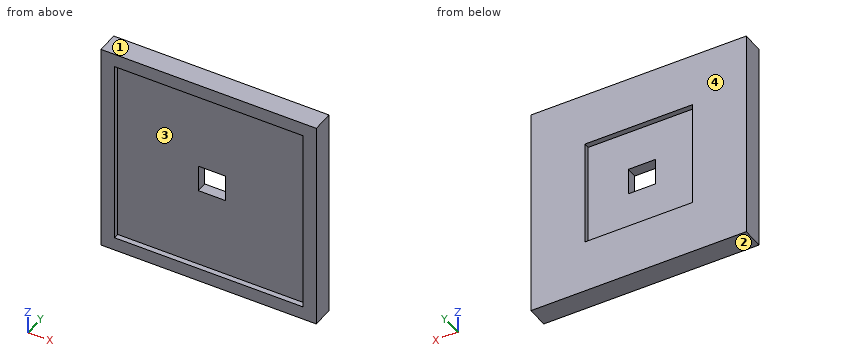
```python
from build123d import *

# Parameters (mm, degrees)
F0_W     = 101.6
F0_H     = 101.6
F1_DEPTH = 10.16
F2_W     = 88.9
F2_H     = 88.9
F3_DEPTH = 2.54
F4_W     = 50.8
F4_H     = 50.8
F5_DEPTH = 2.54
F6_W     = 12.7
F6_H     = 12.7
F7_DEPTH = 25.4


with BuildPart() as f1:
    # F0 (on Front) → F1 (new body)
    with BuildSketch(Plane.XZ):
        with Locations((4.06957, 6.01474)):
            Rectangle(F0_W, F0_H)
    extrude(amount=F1_DEPTH)

    # F2 (on face) → F3 (cut)
    with BuildSketch(Plane.XZ.offset(10.16)):
        with Locations((4.06957, 6.01474)):
            Rectangle(F2_W, F2_H)
    extrude(amount=-F3_DEPTH, mode=Mode.SUBTRACT)

    # F4 (on face) → F5 (cut)
    with BuildSketch(Plane(origin=(0, 0, 0), x_dir=(-1, 0, 0), z_dir=(0, 1, 0))):
        with Locations((-4.06957, 6.01474)):
            Rectangle(F4_W, F4_H)
    extrude(amount=-F5_DEPTH, mode=Mode.SUBTRACT)

    # F6 (on face) → F7 (cut)
    with BuildSketch(Plane(origin=(0, -2.54, 0), x_dir=(-1, 0, 0), z_dir=(0, 1, 0))):
        with Locations((-4.06957, 6.01474)):
            Rectangle(F6_W, F6_H)
    extrude(amount=-F7_DEPTH, mode=Mode.SUBTRACT)


solid = f1.part
```
The listing builds one solid part. Answer for the finished solid, in the listing's coordinates (mm). Face numbers are marked on the shaded views. Give positions to 0.01 mm unless a question says otherwise; leave off trailing zeros. Order: outer loops, then holes, each group sorted by start corner. A loop starts at its lowest first (then second) coordinate and runs counter-clockwise, first axis right, second up. Notation, with made-up numbers: M 47.5,61.5 L 101.5,61.5 A16 cw 101.5,83.5 Z; hole C 3.25,38.25 d3. An arc over 180 degrees is marked long. Put each result on its own line as item: value. Start each with the question number.
Item 1: The part is cut by section D-D, the plane x = -14. Determine the outline of the cut face in (y, z).
Item 2: The part is cut by section A-A, the plane y = -6.25. Determine the outline of the cut face in (x, z), and give its area (3 significant figures).
Item 3: For a pull along Z with two mould halves and no side action, classify the marked faces 1, 2, 3 and 4 as +Z half, -Z half, draft (parallel to the pull), parting line (faces both ways), or undercut.
Item 4: A flat-ended cylindrical pin translates along its axis: P1, Ø1.5, axis at x = -35, z = 35.5, coming from the -Y side. Find the tip coordinate at first contact, or state that the pin passes through.
Item 5: Find the intervals of material crossed by line 1 along X through (y, z) = (-8.5, -17.5); line 2 along Z through (x, y) = (32, -7.75); line 3 along X through (y, z) = (-2.25, -16), in increasing order.
Item 6: The part is cut by section B-B, the plane x = 4.5. Determine the outline of the cut face in (y, z), and give its area (3 significant figures).
Item 7: The part is cut by section C-C, the plane z = 22. Determine the outline of the cut face in (x, y).
Answer key:
1. outline: M -10.16,-44.79 L 0,-44.79 L 0,-19.39 L -2.54,-19.39 L -2.54,31.41 L 0,31.41 L 0,56.81 L -10.16,56.81 L -10.16,50.46 L -7.62,50.46 L -7.62,-38.44 L -10.16,-38.44 Z
2. outline: M -46.73,-44.79 L 54.87,-44.79 L 54.87,56.81 L -46.73,56.81 Z; hole M -2.28,-0.34 L 10.42,-0.34 L 10.42,12.36 L -2.28,12.36 Z
2. area: 10,200 mm²
3. face 1: +Z half
3. face 2: -Z half
3. face 3: undercut
3. face 4: draft
4. P1: stops at y = -7.62
5. line 1: x = -46.73 to -40.38, 48.52 to 54.87
5. line 2: z = -44.79 to -38.44, 50.46 to 56.81
5. line 3: x = -46.73 to -21.33, 29.47 to 54.87
6. outline: M -10.16,-44.79 L 0,-44.79 L 0,-19.39 L -2.54,-19.39 L -2.54,-0.34 L -7.62,-0.34 L -7.62,-38.44 L -10.16,-38.44 Z; M -10.16,50.46 L -7.62,50.46 L -7.62,12.36 L -2.54,12.36 L -2.54,31.41 L 0,31.41 L 0,56.81 L -10.16,56.81 Z
6. area: 613 mm²
7. outline: M -46.73,-10.16 L -40.38,-10.16 L -40.38,-7.62 L 48.52,-7.62 L 48.52,-10.16 L 54.87,-10.16 L 54.87,0 L 29.47,0 L 29.47,-2.54 L -21.33,-2.54 L -21.33,0 L -46.73,0 Z
